Verification items for the finished model (mm, model axes). A direction names the side the tool comes from. Coordinates: 2 decimals unless noted, no trailing zeros. Loops run counter-clockwise (first coordinate to the right, second up) from the corner with the lowest first, then second, coordinate; pieces in that order, holes last. Notation, with made-up numbers: (21.25, 89) -> (49.25, 89) arc R20 cw to (49.25, 113) -> close; hole circle Ø1 at (39, 10.25). An arc over 180 degrees is marked (long way). Write item = value, one per line.
```python
from build123d import *

# Parameters (mm, degrees)
SKETCH1_R           = 1.75
BOSS_EXTRUDE2_DEPTH = 4
SKETCH2_R           = 1.3
CUT_EXTRUDE1_DEPTH  = 10


with BuildPart() as part:
    # Sketch1 → Boss-Extrude2 (new body)
    # profile 1 of 12: a face of its own
    with BuildSketch(Plane.XY):
        with BuildLine():
            Line((30.5, -4), (11.419719786, -4))
            ThreePointArc((11.419719786, -4), (-12.1, 0), (11.419719786, 4))
            Line((11.419719786, 4), (30.5, 4))
            ThreePointArc((30.5, 4), (34.5, 0), (30.5, -4))
        make_face()
        Circle(SKETCH1_R, mode=Mode.SUBTRACT)
        with Locations((30.5, 0)):
            Circle(SKETCH1_R, mode=Mode.SUBTRACT)
    # profile 2 of 12: a face of its own
    with BuildSketch(Plane.XY):
        with BuildLine():
            ThreePointArc((2.04630572, 11.925713098), (3.062574606, 11.706008576), (4.056229837, 11.399868399))
            ThreePointArc((4.056229837, 11.399868399), (4.191789848, 12.739862338), (4.004557713, 14.073618088))
            Line((4.004557713, 14.073618088), (3.400741544, 14.231598069))
            ThreePointArc((3.400741544, 14.231598069), (2.585583316, 13.159679272), (2.04630572, 11.925713098))
        make_face()
    # profile 3 of 12: a face of its own
    with BuildSketch(Plane.XY):
        with BuildLine():
            ThreePointArc((-0.641917286, 12.082960821), (0.397776079, 12.093459976), (1.434532317, 12.014662585))
            ThreePointArc((1.434532317, 12.014662585), (1.27037575, 13.351454601), (0.792800193, 14.610772615))
            Line((0.792800193, 14.610772615), (0.168997044, 14.631297504))
            ThreePointArc((0.168997044, 14.631297504), (-0.388904138, 13.405638858), (-0.641917286, 12.082960821))
        make_face()
    # profile 4 of 12: a face of its own
    with BuildSketch(Plane.XY):
        with BuildLine():
            ThreePointArc((-3.071117398, 14.306350498), (-3.344130279, 12.987655382), (-3.298347959, 11.641773952))
            ThreePointArc((-3.298347959, 11.641773952), (-2.286723162, 11.881956791), (-1.258213497, 12.034404796))
            ThreePointArc((-1.258213497, 12.034404796), (-1.713956435, 13.301787393), (-2.458222459, 14.424297241))
            Line((-2.458222459, 14.424297241), (-3.071117398, 14.306350498))
        make_face()
    # profile 5 of 12: a face of its own
    with BuildSketch(Plane.XY):
        with BuildLine():
            ThreePointArc((-6.159128153, 13.272850751), (-6.133731183, 11.926430371), (-5.791420864, 10.624003218))
            ThreePointArc((-5.791420864, 10.624003218), (-4.857967527, 11.08197417), (-3.888643585, 11.458117257))
            ThreePointArc((-3.888643585, 11.458117257), (-4.613401246, 12.593320589), (-5.587496363, 13.523427559))
            Line((-5.587496363, 13.523427559), (-6.159128153, 13.272850751))
        make_face()
    # profile 6 of 12: a face of its own
    with BuildSketch(Plane.XY):
        with BuildLine():
            ThreePointArc((-8.942094855, 11.581984556), (-8.619545875, 10.274523276), (-7.997661209, 9.080055902))
            ThreePointArc((-7.997661209, 9.080055902), (-7.188610613, 9.733132972), (-6.326480245, 10.314341845))
            ThreePointArc((-6.326480245, 10.314341845), (-7.28435745, 11.261142529), (-8.440037507, 11.952781076))
            Line((-8.440037507, 11.952781076), (-8.942094855, 11.581984556))
        make_face()
    # profile 7 of 12: a face of its own
    with BuildSketch(Plane.XY):
        with BuildLine():
            ThreePointArc((-11.2821851, 9.317495695), (-10.67845904, 8.113748343), (-9.807800202, 7.086399311))
            ThreePointArc((-9.807800202, 7.086399311), (-9.163222316, 7.902237454), (-8.450984381, 8.659726496))
            ThreePointArc((-8.450984381, 8.659726496), (-9.594540202, 9.371232193), (-10.874567661, 9.790147432))
            Line((-10.874567661, 9.790147432), (-11.2821851, 9.317495695))
        make_face()
    # profile 8 of 12: a face of its own
    with BuildSketch(Plane.XY):
        with BuildLine():
            ThreePointArc((-13.06350089, 6.591537844), (-12.208498581, 5.551122593), (-11.13218682, 4.741773571))
            ThreePointArc((-11.13218682, 4.741773571), (-10.684005749, 5.67996665), (-10.15693536, 6.576219589))
            ThreePointArc((-10.15693536, 6.576219589), (-11.42953274, 7.017191451), (-12.770511491, 7.142635705))
            Line((-12.770511491, 7.142635705), (-13.06350089, 6.591537844))
        make_face()
    # profile 9 of 12: a face of its own
    with BuildSketch(Plane.XY):
        with BuildLine():
            ThreePointArc((4.633181039, 11.177818815), (5.575692546, 10.738791954), (6.47703386, 10.22047124))
            ThreePointArc((6.47703386, 10.22047124), (6.905596548, 11.497301024), (7.017980909, 12.839437391))
            Line((7.017980909, 12.839437391), (6.464057014, 13.127048167))
            ThreePointArc((6.464057014, 13.127048167), (5.432014202, 12.2619583), (4.633181039, 11.177818815))
        make_face()
    # profile 10 of 12: a face of its own
    with BuildSketch(Plane.XY):
        with BuildLine():
            ThreePointArc((6.990588114, 9.876319042), (7.812662335, 9.239713591), (8.577048867, 8.534883288))
            ThreePointArc((8.577048867, 8.534883288), (9.277388744, 9.685311177), (9.683823524, 10.969355975))
            Line((9.683823524, 10.969355975), (9.207226173, 11.372353004))
            ThreePointArc((9.207226173, 11.372353004), (8.009412915, 10.7569375), (6.990588114, 9.876319042))
        make_face()
    # profile 11 of 12: a face of its own
    with BuildSketch(Plane.XY):
        with BuildLine():
            ThreePointArc((9.001771295, 8.085673352), (9.662693238, 7.283018563), (10.252267103, 6.426586905))
            ThreePointArc((10.252267103, 6.426586905), (11.189698333, 7.393635488), (11.870053976, 8.555993639))
            Line((11.870053976, 8.555993639), (11.494387677, 9.054417628))
            ThreePointArc((11.494387677, 9.054417628), (10.190128247, 8.719156263), (9.001771295, 8.085673352))
        make_face()
    # profile 12 of 12: a face of its own
    with BuildSketch(Plane.XY):
        with BuildLine():
            ThreePointArc((10.567122415, 5.894567319), (11.034158501, 4.965616394), (11.419719786, 4))
            ThreePointArc((11.419719786, 4), (12.547814073, 4.735774119), (13.468394505, 5.718877338))
            Line((13.468394505, 5.718877338), (13.212264939, 6.288042768))
            ThreePointArc((13.212264939, 6.288042768), (11.866155587, 6.249540081), (10.567122415, 5.894567319))
        make_face()
    extrude(amount=BOSS_EXTRUDE2_DEPTH)

    # Sketch2 → Cut-Extrude1 (cut)
    with BuildSketch(Plane(origin=(0, 0, 0), x_dir=(-1, 0, 0), z_dir=(0, 0, -1))):
        with Locations((4.5, 0)):
            Circle(SKETCH2_R)
        with Locations((-4.5, 0)):
            Circle(SKETCH2_R)
    extrude(amount=-CUT_EXTRUDE1_DEPTH, mode=Mode.SUBTRACT)


solid = part.part
```
1) Sectioned sample at D-D, the plane x = 23.5. Record the cut outline in (y, z), plus the area to 3 significant figures.
Ans:
outline = (-4, 0) -> (4, 0) -> (4, 4) -> (-4, 4) -> close
area = 32.0 mm2
2) Sectioned sample at C-C, the plane z = 2.8. Count the separate pieces of the cut face and the enclosed holes in it, plus the area to 3 significant figures.
Ans:
separate_pieces = 1
enclosed_holes = 4
area = 648 mm2
3) Depth check by flat-ended pin: pin 1 Ø1 at (x, z) = (16.5, 1) entering from -Y; pin 2 Ø1 at (x, z) = (2.5, 2.5) entering from -Y. Enter the tip coordinate at first touch or a pass-through.
Ans:
pin_1 = -4
pin_2 = -11.93
4) Sectioned sample at B-B, the plane x = -4.5. Record the cut outline in (y, z), plus the area to 3 significant figures.
Ans:
outline = (-11.23, 0) -> (-1.3, 0) -> (-1.3, 4) -> (-11.23, 4) -> close; (1.3, 0) -> (12.45, 0) -> (12.45, 4) -> (1.3, 4) -> close
area = 84.3 mm2
5) Tool access check on faces 5 (the face through (5.445, 12.276, 1.972)), 6 (the face through (5.1, 1.5, 0)), 7 (the face through (6.9, 11.48, 1.97)). Record the directions out of +Z, -Z, +X, -X, +Y, -Y that give a thin tool (end or side, any length) a straight path to the whole face; none if there is none.
Ans:
face_5 = +Z, -Z, +Y
face_6 = -Z, +X, -X, +Y, -Y
face_7 = +Z, -Z
6) Sectioned sample at A-A, the plane y = 0. Record the cut outline in (x, z).
Ans:
outline = (-12.1, 0) -> (-5.8, 0) -> (-5.8, 4) -> (-12.1, 4) -> close; (-3.2, 0) -> (-1.75, 0) -> (-1.75, 4) -> (-3.2, 4) -> close; (1.75, 0) -> (3.2, 0) -> (3.2, 4) -> (1.75, 4) -> close; (5.8, 0) -> (28.75, 0) -> (28.75, 4) -> (5.8, 4) -> close; (32.25, 0) -> (34.5, 0) -> (34.5, 4) -> (32.25, 4) -> close
7) Material ranges on line 1 (Y direction, x = 30.5, z = 2.25); line 2 (Y direction, x = 13, z = 1.3); line 3 (X direction, y = 8.5, z = 2.1), recorded low to high.
Ans:
line_1 = -4 to -1.75, 1.75 to 4
line_2 = -4 to 4, 5.16 to 6.3
line_3 = -10.91 to 8.61, 9.7 to 11.85
8) Release check for a two-part mould opening along X. For faces 1 (the face through (21, 4, 2)), 2 (the face through (-12.22, 5.56, 1.97)), 3 (the face through (34.5, 0.1, 2)), 4 (the face through (-1.706, 13.285, 1.972)) record: pulls with the +X half, pulls with the -X half, needs draft (parallel to the pull), parting line crosses it, or undercut.
Ans:
face_1 = needs draft
face_2 = pulls with the -X half
face_3 = pulls with the +X half
face_4 = undercut
